The drawing under review shows one solid part. Ordinate dimensions are in mm from its lowest x, y, z. A direction names the side the tool comes from. Coordinates: 2 decimals unless noted, no trailing zeros. Order: outer loops, then holes, each group sorted by start corner. A loop starts at its lowest first (then second) coordinate and runs counter-clockwise, first axis right, second up. Notation, with made-up numbers: M -30.75,-30 L 5.25,-30 A35 cw 5.25,4 Z; hole C 31,-26 d3. An arc over 180 degrees is marked long. Answer as a JSON object with one key per item and string values.
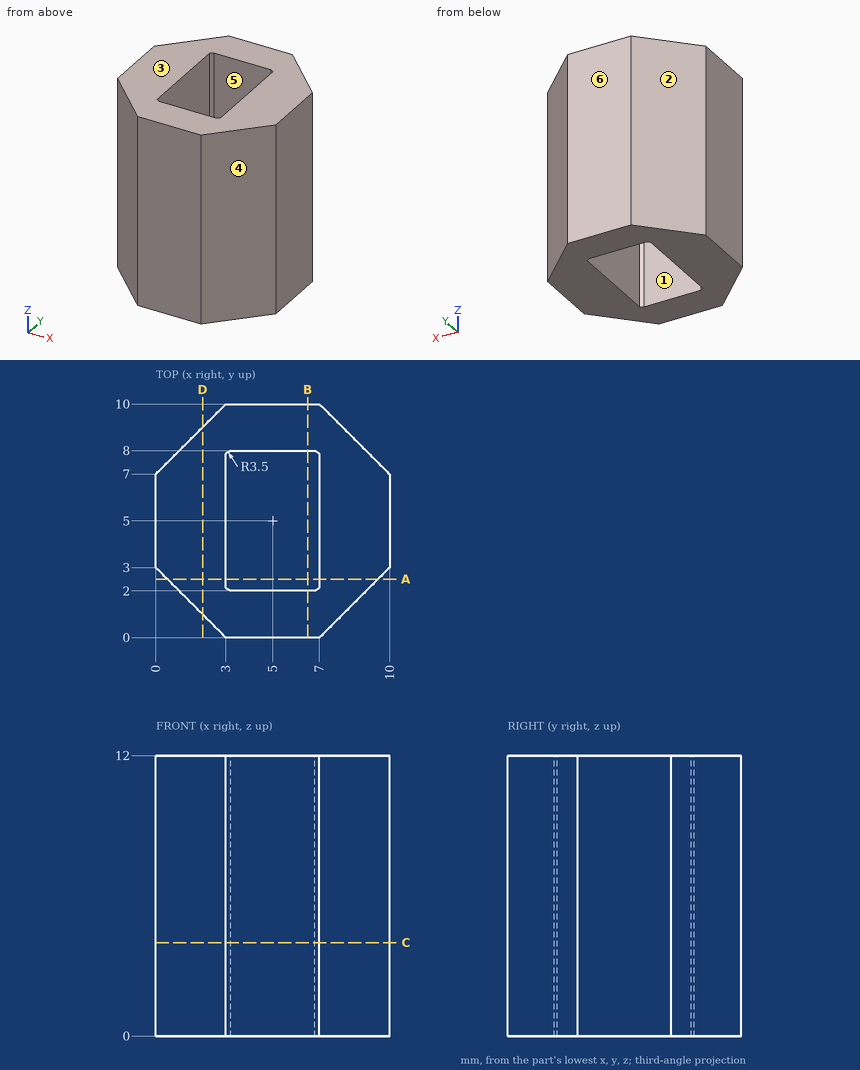
1) To check wall thickness, follow L1, parallel to X at y = 5.75, z = 9.5; L2, parallel to Y at x = 6, z = 1.5; L3, parallel to X at y = 2.5, z = 9.25. State the ranges of each line that lie inside material, in increasing order.
Taken from the geometry:
{"L1": "x = 0 to 3, 7 to 10", "L2": "y = 0 to 2, 8 to 10", "L3": "x = 0.5 to 3, 7 to 9.5"}
2) Add section A-A (y = 2.5). State the section outline as (x, z) points.
Taken from the geometry:
{"outline": "M 0.5,0 L 3,0 L 3,12 L 0.5,12 Z; M 7,0 L 9.5,0 L 9.5,12 L 7,12 Z"}
3) Tool access review of the marked faces 5 and 6: name each direction out of +Z, -Z, +X, -X, +Y, -Y from which nothing blocks a thin tool from reaching the whole face with its end or side.
Taken from the geometry:
{"face 5": "+Z, -Z", "face 6": "+Z, -Z, +X, -X, +Y"}
4) Add section C-C (z = 4). State the section outline as (x, y) points, and give its area (3 significant figures).
Taken from the geometry:
{"outline": "M 0,3 L 3,0 L 7,0 L 10,3 L 10,7 L 7,10 L 3,10 L 0,7 Z; hole M 3,2.13 A3.5 ccw 3.2,2 L 6.8,2 A3.5 ccw 7,2.13 L 7,7.87 A3.5 ccw 6.8,8 L 3.2,8 A3.5 ccw 3,7.87 Z", "area": "58.0 mm2"}
5) Add section D-D (x = 2). State the section outline as (y, z) points, and give its area (3 significant figures).
Taken from the geometry:
{"outline": "M 1,0 L 9,0 L 9,12 L 1,12 Z", "area": "96.0 mm2"}
6) Mouldability with a two-part tool opening along X and no side actions: class the marked faces 1, 2, 3 and 4 as released by +X, released by -X, zero draft, split by the parting line, or undercut.
Taken from the geometry:
{"face 1": "undercut", "face 2": "released by -X", "face 3": "zero draft", "face 4": "released by +X"}
7) Add section B-B (x = 6.5). State the section outline as (y, z) points, and give its area (3 significant figures).
Taken from the geometry:
{"outline": "M 0,0 L 2,0 L 2,12 L 0,12 Z; M 8,0 L 10,0 L 10,12 L 8,12 Z", "area": "48.0 mm2"}
